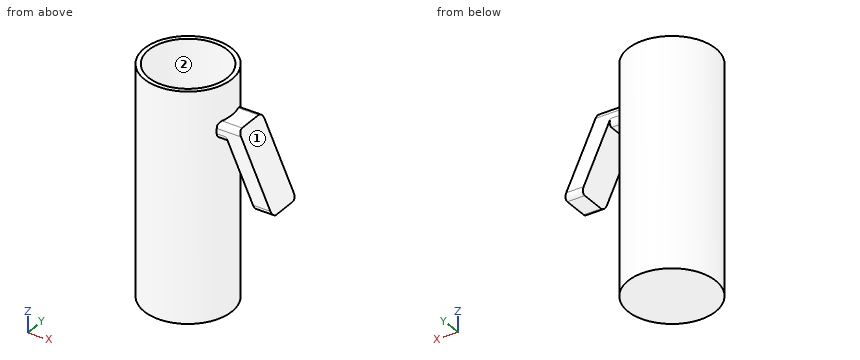
from build123d import *

# Parameters (mm, degrees)
F0_W      = 2.54
F0_H      = 11.43
F2_DEPTH  = 12.7
F3_R      = 3.81
F4_R      = 28.575
F5_DEPTH  = 76.2
F5_FACE_R = 28.575
F6_DEPTH  = 78.74


with BuildPart() as f1:
    # F0 (on Front) → F1 (revolve)
    with BuildSketch(Plane.XZ):
        Polygon((31.75, 0), (0, 0), (0, -165.1), (31.75, -165.1), (31.75, -36.83), (29.21, -36.83), (29.21, -25.4), (31.75, -25.4), align=None)
        with Locations((30.48, -31.115)):
            Rectangle(F0_W, F0_H)
    revolve(axis=Axis((0, 0, -82.55), (0, 0, -1)))

    # F0 (on Front) → F2 (join, symmetric)
    with BuildSketch(Plane.XZ):
        Polygon((45.085, -25.4), (31.75, -25.4), (31.75, -36.83), (37.803287, -36.83), (57.23839, -78.508714), (69.85, -78.508714), align=None)
        with Locations((30.48, -31.115)):
            Rectangle(F0_W, F0_H)
    extrude(amount=F2_DEPTH, both=True)

    # F3
    f3_edges = [f1.edges().sort_by_distance(p)[0] for p in [
        (37.1475, -12.7, -25.4),
        (37.1475, 12.7, -25.4),
        (33.506643, 12.7, -36.83),
        (33.506643, -12.7, -36.83),
        (63.544195, -12.7, -78.508714),
        (63.544195, 12.7, -78.508714),
    ]]
    fillet(f3_edges, radius=F3_R)

    # F4 (on face) → F5 (cut)
    with BuildSketch(Plane.XY):
        Circle(F4_R)
    extrude(amount=-F5_DEPTH, mode=Mode.SUBTRACT)

    # F5_face (on face) → F6 (cut)
    with BuildSketch(Plane.XY.offset(-76.2)):
        Circle(F5_FACE_R)
    extrude(amount=-F6_DEPTH, mode=Mode.SUBTRACT)


solid = f1.part
Check sheet for the modelled part. Datum: model origin and axes. Units: mm. Face numbers are marked on the shaded views. A direction names the side the tool comes from. Round coordinates to 2 decimals unless told otherwise and drop trailing zeros. Loops run counter-clockwise (first coordinate to the right, second up) from the corner with the lowest first, then second, coordinate; pieces in that order, holes last. Notation, with made-up numbers: (-7, -28.75) -> (50, -28.75) arc R15 cw to (50, -5.75) -> close; hole circle Ø11 at (25.25, -32.75). An arc over 180 degrees is marked (long way). Put each result on its own line as item: value. Start each with the question number.
1. Section check D-D (z = -90). Enter the section's corners in (x, y) (3 decimals).
2. Section check B-B (x = 0). Enter the section's corners in (y, z) (3 decimals).
3. Access from +Z, -Z, +X, -X, +Y, -Y to the whole of each face (thin tool, end or side, straight path). Record for the marked faces 1 and 2.
4. Scan lines: probe 1 along Y at (x, z) = (0, -91) (3 decimals); probe 2 along X at (y, z) = (-3, -43); probe 3 along X at (y, z) = (7.5, -61.5). Record each from-to range of solid material in increasing order.
5. Section check C-C (y = 4). Enter the section's corners in (x, z) (3 decimals).
6. Gauge pin test, flat ends, axial feed: pin 1 (6 mm diameter, centred on x = 15.5, z = -75, fed in from -Y); pin 2 (6 mm diameter, centred on x = 49.5, z = -39, fed in from +Y); pin 3 (10 mm diameter, centred on y = 9, z = -25, fed in from +X). Record the tip position at first contact, or that the pin passes through.
7. Section check A-A (z = -52). Enter the section's corners in (x, y) (3 decimals), plus the area to 3 significant figures.
Findings:
1. outline: circle Ø63.5 at (0, 0); hole circle Ø57.15 at (0, 0)
2. outline: (-31.75, -165.1) -> (31.75, -165.1) -> (31.75, 0) -> (28.575, 0) -> (28.575, -154.94) -> (-28.575, -154.94) -> (-28.575, 0) -> (-31.75, 0) -> close
3. face 1: +Z, +X, +Y, -Y
3. face 2: +Z
4. probe 1: y = -31.75 to -28.575, 28.575 to 31.75
4. probe 2: x = -31.61 to -28.42, 28.42 to 31.61, 40.68 to 53.29
4. probe 3: x = -30.85 to -27.57, 27.57 to 30.85, 49.31 to 61.92
5. outline: (-31.497, -165.1) -> (31.497, -165.1) -> (31.497, -36.83) -> (37.803, -36.83) -> (57.238, -78.509) -> (69.85, -78.509) -> (45.085, -25.4) -> (31.497, -25.4) -> (31.497, 0) -> (28.294, 0) -> (28.294, -154.94) -> (-28.294, -154.94) -> (-28.294, 0) -> (-31.497, 0) -> close
6. pin 1: stops at y = -29.19
6. pin 2: stops at y = 12.7
6. pin 3: stops at x = 47.23
7. outline: circle Ø63.5 at (0, 0); (44.877, -12.7) -> (57.489, -12.7) -> (57.489, 12.7) -> (44.877, 12.7) -> close; hole circle Ø57.15 at (0, 0)
7. area: 922 mm^2
